```python
from build123d import *

# Parameters (mm, degrees)
SKETCH1_R           = 11
SKETCH1_R_2         = 5
SKETCH1_R_3         = 1.5
BOSS_EXTRUDE1_DEPTH = 5
SKETCH2_W           = 5
SKETCH2_H           = 65
BOSS_EXTRUDE2_DEPTH = 25
SKETCH3_W           = 72.3
SKETCH3_H           = 65
BOSS_EXTRUDE3_DEPTH = 5
SKETCH4_W           = 65
SKETCH4_H           = 75
SKETCH4_R           = 4
BOSS_EXTRUDE4_DEPTH = 5


with BuildPart() as part:
    # Sketch1 → Boss-Extrude1 (new body)
    with BuildSketch(Plane(origin=(0, 0, 0), x_dir=(0, 0, -1), z_dir=(1, 0, 0))):
        Polygon((-17.5, 27.5), (-27.5, 27.5), (-27.5, 17.5), (-27.5, -27.5), (37.5, -27.5), (37.5, 7.5), (37.5, 27.5), (17.5, 27.5), align=None)
        with Locations((5, 0)):
            Circle(SKETCH1_R, mode=Mode.SUBTRACT)
        with Locations((5, 17.5)):
            Circle(SKETCH1_R_2, mode=Mode.SUBTRACT)
        with Locations((30, 17.5)):
            Circle(SKETCH1_R_3, mode=Mode.SUBTRACT)
        with Locations((-20, 17.5)):
            Circle(SKETCH1_R_3, mode=Mode.SUBTRACT)
    extrude(amount=BOSS_EXTRUDE1_DEPTH)

    # Sketch2 → Boss-Extrude2 (add)
    with BuildSketch(Plane.XZ.offset(27.5)):
        with Locations((2.5, -5)):
            Rectangle(SKETCH2_W, SKETCH2_H)
    extrude(amount=BOSS_EXTRUDE2_DEPTH)

    # Sketch3 → Boss-Extrude3 (add)
    with BuildSketch(Plane.XZ.offset(52.5)):
        with Locations((-36.15, -5)):
            Rectangle(SKETCH3_W, SKETCH3_H)
    extrude(amount=-BOSS_EXTRUDE3_DEPTH)

    # Sketch4 → Boss-Extrude4 (add)
    with BuildSketch(Plane.ZY.offset(72.3)):
        with Locations((-5, -10)):
            Rectangle(SKETCH4_W, SKETCH4_H)
        with Locations((-5, 0)):
            Circle(SKETCH4_R, mode=Mode.SUBTRACT)
    extrude(amount=-BOSS_EXTRUDE4_DEPTH)


solid = part.part
```
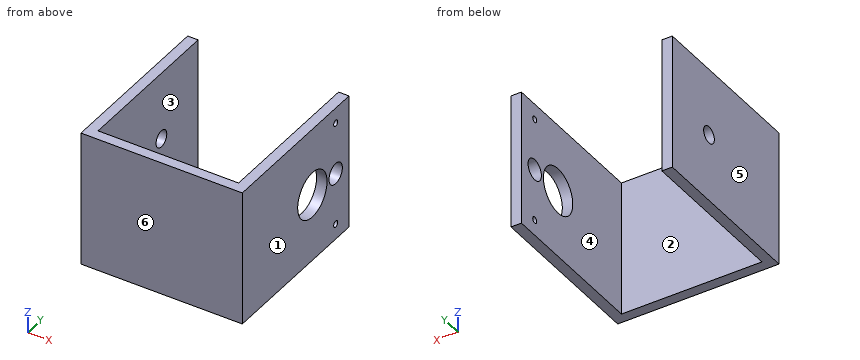
Build history of the part. All positions in model axes, mm. Face numbers are marked on the shaded views. A direction names the side the tool comes from. Round coordinates to 2 decimals unless told otherwise and drop trailing zeros. Order: outer loops, then holes, each group sorted by start corner. A loop starts at its lowest first (then second) coordinate and runs counter-clockwise, first axis right, second up. Notation, with made-up numbers: (20.5, 88.5) - (57.5, 88.5) arc R13 cw to (57.5, 111.5) - close; hole circle Ø2 at (3.25, 33.25). An arc over 180 degrees is marked (long way). Use a Markdown table: item, result.
1) Wall check: L1, parallel to Y at x = 2.4, z = -5; L2, parallel to X at y = -29, z = -2; L3, parallel to Y at x = 3, z = -30. Give the ranges that are in metal, low to high.
Recorded:
| item | result |
|---|---|
| L1 | y = -52.5 to -11, 11 to 12.5, 22.5 to 27.5 |
| L2 | x = -72.3 to -67.3, 0 to 5 |
| L3 | y = -52.5 to 16, 19 to 27.5 |
2) Saw through at C-C on y = -22.5. Write the cut outline in (x, z), and give its area (3 significant figures).
Recorded:
| item | result |
|---|---|
| outline | (-72.3, -37.5) - (-67.3, -37.5) - (-67.3, 27.5) - (-72.3, 27.5) - close; (0, -37.5) - (5, -37.5) - (5, 27.5) - (0, 27.5) - close |
| area | 650 mm² |
3) Flat gauge pins, fed straight in: pin 1 Ø2 at (x, z) = (-33, 18) entering from +Y; pin 2 Ø19.5 at (y, z) = (7.5, 1.5) entering from +X; pin 3 Ø7 at (y, z) = (0, -5) entering from +X; pin 4 Ø6 at (y, z) = (17.5, -5) entering from +X. Where does each tip first touch, or does it go through?
Recorded:
| item | result |
|---|---|
| pin 1 | stops at y = -47.5 |
| pin 2 | stops at x = 5 |
| pin 3 | passes through |
| pin 4 | stops at x = -67.3 |
4) Saw through at D-D on x = -4. Write the cut outline in (y, z), and give its area (3 significant figures).
Recorded:
| item | result |
|---|---|
| outline | (-52.5, -37.5) - (-47.5, -37.5) - (-47.5, 27.5) - (-52.5, 27.5) - close |
| area | 325 mm² |
5) Tool access for the marked faces 1 and 2: list every direction of +Z, -Z, +X, -X, +Y, -Y with a clear straight run to the whole face (end or side of a thin tool).
Recorded:
| item | result |
|---|---|
| face 1 | +Z, -Z, +X, +Y, -Y |
| face 2 | +Z, -Z, +Y |
6) Saw through at B-B on z = -30. Write the cut outline in (x, y).
Recorded:
| item | result |
|---|---|
| outline | (-72.3, -52.5) - (5, -52.5) - (5, 16) - (0, 16) - (0, -47.5) - (-67.3, -47.5) - (-67.3, 27.5) - (-72.3, 27.5) - close; (0, 19) - (5, 19) - (5, 27.5) - (0, 27.5) - close |
7) Pull direction X, two halves, no side cores. Call the marked faces 3, 4, 5 and 6: pulls with the +X half, pulls with the -X half, needs draft (parallel to the pull), parting line crosses it, or undercut.
Recorded:
| item | result |
|---|---|
| face 3 | undercut |
| face 4 | undercut |
| face 5 | pulls with the -X half |
| face 6 | needs draft |
8) Saw through at A-A on y = 0. Write the cut outline in (x, z), and give its area (3 significant figures).
Recorded:
| item | result |
|---|---|
| outline | (-72.3, -37.5) - (-67.3, -37.5) - (-67.3, -9) - (-72.3, -9) - close; (-72.3, -1) - (-67.3, -1) - (-67.3, 27.5) - (-72.3, 27.5) - close; (0, -37.5) - (5, -37.5) - (5, -16) - (0, -16) - close; (0, 6) - (5, 6) - (5, 27.5) - (0, 27.5) - close |
| area | 500 mm² |
